Read the model definition and answer for the solid it produces. Units are mm, in the model's axes. Face numbers are marked on the shaded views. A direction names the side the tool comes from. Coordinates: 2 decimals unless noted, no trailing zeros. Write each loop counter-clockwise with the first axis right and the second up, starting at its lowest first coordinate (ties: lowest second). Pieces come first, ordered by that corner, then holes.
1) The part is cut by section D-D (x = 75). Give the number of separate pieces and of enclosed holes in the cut face, then the cut area to 3 significant figures.
2) Which of the six approach directions +Z, -Z, +X, -X, +Y, -Y give full straight-line access (tool end or side, diameter ignored) to the marked faces 1, 2, 3, 4 and 5?
3) Each of these flat-tipped pins is pushed along its axis until it touches: pin 1 Ø10 at (x, z) = (50, 13.5) entering from +Y; pin 2 Ø6 at (y, z) = (3.5, 12) entering from +X; pin 3 Ø1 at (x, z) = (-8.5, 14.5) entering from +Y. Where does it stop, or does it pass through?
4) The part is cut by section B-B (y = 21). Determine the outline of the cut face in (x, z), then the cut area to 3 significant figures.
5) Find the intervals of material crossed by line 1 (Y direction, x = 75, z = 17.6); line 2 (X direction, y = 6, z = 8.25); line 3 (Y direction, x = 62, z = 10.5), in increasing order.
6) Determine the mould class of the marked faces 6, 7, 8 and 9 for opening direction Y: +Y half, -Y half, draft (parallel to the pull), parting line (faces both ways), or undercut.
7) The part is cut by section A-A (x = -12.5). Determine the outline of the cut face in (y, z).
8) The part is cut by section C-C (y = 0). Determine the outline of the cut face in (x, z), then the cut area to 3 significant figures.
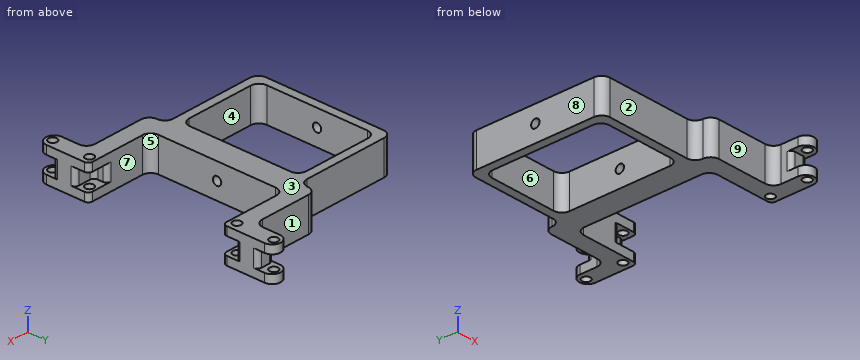
from build123d import *

# Parameters (mm, degrees)
SKETCH1_W           = 60
SKETCH1_H           = 80
SKETCH1_W_2         = 50
SKETCH1_H_2         = 70
EXTRUDE_THIN2_DEPTH = 20
EXTRUDE_THIN4_START = -20
EXTRUDE_THIN4_DEPTH = 20
SKETCH3_R           = 2.5
CUT_EXTRUDE1_DEPTH  = 115.891252931
SKETCH4_W           = 17.535354843
SKETCH4_H           = 20
CUT_EXTRUDE2_DEPTH  = 115.891252931
FILLET1_RADIUS      = 5
FILLET1_LENGTH      = 20
SKETCH5_W           = 12
SKETCH5_H           = 8
SKETCH5_W_2         = 13.595286796
SKETCH5_H_2         = 19.881342556
CUT_EXTRUDE3_DEPTH  = 5
FILLET2_RADIUS      = 5
FILLET2_LENGTH      = 20
SKETCH6_R           = 2.5
CUT_EXTRUDE4_DEPTH  = 102.004981635
FILLET3_R           = 5
FILLET4_R           = 2.5


# Read off the part's stored shape, not the designer's step: Extrude-Thin4
with BuildPart() as part:
    # Sketch1 → Extrude-Thin2 (new body)
    with BuildSketch(Plane.XY):
        Rectangle(SKETCH1_W, SKETCH1_H)
        Rectangle(SKETCH1_W_2, SKETCH1_H_2, mode=Mode.SUBTRACT)
    extrude(amount=EXTRUDE_THIN2_DEPTH)

    # Extrude-Thin4 outline → Extrude-Thin4 (add)
    with BuildSketch(Plane.XY.offset(20).offset(EXTRUDE_THIN4_START)):
        Polygon((70, 50), (30, 50), (30, -50), (70, -50), (70, -80), (80, -80), (80, -40), (40, -40), (40, 40), (80, 40), (80, 80), (70, 80), align=None)
    extrude(amount=EXTRUDE_THIN4_DEPTH)

    # Sketch3 → Cut-Extrude1 (cut, through all)
    with BuildSketch(Plane.XY.offset(20)):
        with Locations((75, -66.014329355)):
            Circle(SKETCH3_R)
        with Locations((75, -44.014329355)):
            Circle(SKETCH3_R)
    cut_extrude1 = extrude(amount=-CUT_EXTRUDE1_DEPTH, mode=Mode.SUBTRACT)

    # Sketch4 → Cut-Extrude2 (cut, through all)
    with BuildSketch(Plane.XY.offset(20)):
        with Locations((73.91933671, -80.014329355)):
            Rectangle(SKETCH4_W, SKETCH4_H)
    cut_extrude2 = extrude(amount=-CUT_EXTRUDE2_DEPTH, mode=Mode.SUBTRACT)

    # Fillet1: full round fillet: the end face becomes a half cylinder, R = half its width
    fillet1_face = Plane((75, -70.014329355, 10), x_dir=(0, 0, 1), z_dir=(0, -1, 0))  # on the end face: x along it, z out of the body
    fillet1_slab = fillet1_face.offset(-FILLET1_RADIUS / 2) * Box(FILLET1_LENGTH, 2 * FILLET1_RADIUS, FILLET1_RADIUS, mode=Mode.PRIVATE)  # the body's end, R deep
    fillet1_round = Plane((75, -65.014329355, 10), x_dir=(0, -1, 0), z_dir=(0, 0, 1)) * Cylinder(FILLET1_RADIUS, FILLET1_LENGTH, mode=Mode.PRIVATE)  # its axis R under the face
    add(fillet1_slab - fillet1_round, mode=Mode.SUBTRACT)

    # Sketch5 → Cut-Extrude3 (cut, symmetric)
    with BuildSketch(Plane.XY.offset(10)):
        with Locations((74, -44)):
            Rectangle(SKETCH5_W, SKETCH5_H)
        with Locations((75.604543017, -70.955000633)):
            Rectangle(SKETCH5_W_2, SKETCH5_H_2)
    cut_extrude3 = extrude(amount=CUT_EXTRUDE3_DEPTH, both=True, mode=Mode.SUBTRACT)

    # Mirror6: Cut-Extrude1 across plane
    add(cut_extrude1.mirror(Plane(origin=(0, 0, 0), x_dir=(0, 0, 1), z_dir=(0, -1, 0))), mode=Mode.SUBTRACT)

    # Mirror8: Cut-Extrude2 across plane
    add(cut_extrude2.mirror(Plane(origin=(0, 0, 0), x_dir=(0, 0, 1), z_dir=(0, -1, 0))), mode=Mode.SUBTRACT)

    # Fillet2: full round fillet: the end face becomes a half cylinder, R = half its width
    fillet2_face = Plane((75, 70.014329355, 10), x_dir=(0, 0, -1), z_dir=(0, 1, 0))  # on the end face: x along it, z out of the body
    fillet2_slab = fillet2_face.offset(-FILLET2_RADIUS / 2) * Box(FILLET2_LENGTH, 2 * FILLET2_RADIUS, FILLET2_RADIUS, mode=Mode.PRIVATE)  # the body's end, R deep
    fillet2_round = Plane((75, 65.014329355, 10), x_dir=(0, 1, 0), z_dir=(0, 0, -1)) * Cylinder(FILLET2_RADIUS, FILLET2_LENGTH, mode=Mode.PRIVATE)  # its axis R under the face
    add(fillet2_slab - fillet2_round, mode=Mode.SUBTRACT)

    # Mirror9: Cut-Extrude3 across plane
    add(cut_extrude3.mirror(Plane(origin=(0, 0, 0), x_dir=(0, 0, 1), z_dir=(0, -1, 0))), mode=Mode.SUBTRACT)

    # Sketch6 → Cut-Extrude4 (cut, through all)
    with BuildSketch(Plane(origin=(40, 0, 0), x_dir=(0, 0, -1), z_dir=(1, 0, 0))):
        with Locations((-10, 0)):
            Circle(SKETCH6_R)
    extrude(amount=-CUT_EXTRUDE4_DEPTH, mode=Mode.SUBTRACT)

    # Fillet3
    fillet3_edges = [part.edges().sort_by_distance(p)[0] for p in [
        (-30, -40, 10),
        (70, -50, 10),
        (70, 50, 10),
        (30, 50, 10),
        (30, -50, 10),
        (-25, -35, 10),
        (25, -35, 10),
        (25, 35, 10),
        (-25, 35, 10),
        (30, -40, 10),
        (30, 40, 10),
        (-30, 40, 10),
        (40, -40, 10),
        (40, 40, 10),
    ]]
    fillet(fillet3_edges, radius=FILLET3_R - 0.0001)  # a hair under: the kernel refuses the full size

    # Fillet4
    fillet4_edges = [part.edges().sort_by_distance(p)[0] for p in [
        (80, -40, 17.5),
        (80, -61.014329355, 10),
        (80, -48, 10),
        (68, -40, 10),
        (68, -48, 10),
        (70, -61.014329355, 10),
        (80, 40, 17.5),
        (80, 61.014329355, 10),
        (80, 48, 10),
        (68, 48, 10),
        (68, 40, 10),
        (70, 61.014329355, 10),
        (80, 40, 2.5),
        (80, -40, 2.5),
    ]]
    fillet(fillet4_edges, radius=FILLET4_R)


solid = part.part
Reported:
1. separate pieces: 10
1. enclosed holes: 0
1. area: 661 mm2
2. face 1: +Z, -Z, -X, +Y
2. face 2: +Z, -Z, -X, -Y
2. face 3: +Z, +X, -X, +Y, -Y
2. face 4: +Z, -Z
2. face 5: +Z, -Z, +X
3. pin 1: stops at y = 50
3. pin 2: stops at x = 40
3. pin 3: stops at y = 40
4. outline: (-30, 0) - (-25, 0) - (-25, 20) - (-30, 20) - close; (25, 0) - (40, 0) - (40, 20) - (25, 20) - close
4. area: 400 mm2
5. line 1: y = -70.01 to -68.51, -63.51 to -46.51, -41.51 to -40, 40 to 41.51, 46.51 to 63.51, 68.51 to 70.01
5. line 2: x = -30 to -25, 25 to 40
5. line 3: y = -50 to -40, 40 to 50
6. face 6: undercut
6. face 7: undercut
6. face 8: draft
6. face 9: -Y half
7. outline: (-40, 0) - (-35, 0) - (-35, 20) - (-40, 20) - close; (35, 0) - (40, 0) - (40, 20) - (35, 20) - close
8. outline: (-30, 0) - (-25, 0) - (-25, 7.5) - (-30, 7.5) - close; (-30, 12.5) - (-25, 12.5) - (-25, 20) - (-30, 20) - close; (25, 0) - (40, 0) - (40, 7.5) - (25, 7.5) - close; (25, 12.5) - (40, 12.5) - (40, 20) - (25, 20) - close
8. area: 300 mm2
